```python
from build123d import *

# Parameters (mm, degrees)
SKETCH1_R                = 34.544
BOSS_EXTRUDE1_DEPTH      = 7.62
SKETCH2_R                = 28.1686
CUT_EXTRUDE1_DEPTH       = 3.048
CUT_EXTRUDE2_START       = -1.778
SKETCH3_R                = 28.1686
SKETCH3_R_2              = 4.3688
CUT_EXTRUDE2_DEPTH       = 1.778
CUT_EXTRUDE3_DEPTH       = 50.200658898
FILLET1_R                = 1.6002
CIRPATTERN1_COUNT        = 5
FILLET1_OF_CIRPATTERN1_R = 1.6002
SKETCH5_R                = 17.4625
SKETCH5_R_2              = 10.7061
BOSS_EXTRUDE2_DEPTH      = 1.778
BOSS_EXTRUDE4_START      = 1.6002
SKETCH6_R                = 17.4625
SKETCH6_R_2              = 16.4211
BOSS_EXTRUDE4_DEPTH      = 1.6002
SKETCH7_R                = 3.175
CUT_EXTRUDE4_DEPTH       = 50.066068275
SKETCH8_R                = 1.4224
CUT_EXTRUDE5_DEPTH       = 50.066068275
CIRPATTERN2_COUNT        = 5
BOSS_EXTRUDE5_DEPTH      = 0.0254
BOSS_EXTRUDE5_DEPTH_BACK = 7.6454
SKETCH9_R                = 34.5567
SKETCH9_R_2              = 30.4165
SCALE_1_SCALE            = 3


with BuildPart() as part:
    # Sketch1 → Boss-Extrude1 (new body)
    with BuildSketch(Plane(origin=(0, 0, 0), x_dir=(0, 0, -1), z_dir=(1, 0, 0))):
        with Locations(Location((0, 0, 0), (0, 0, 180))):
            Circle(SKETCH1_R)
    extrude(amount=BOSS_EXTRUDE1_DEPTH)

    # Sketch2 → Cut-Extrude1 (cut)
    with BuildSketch(Plane(origin=(7.62, 0, 0), x_dir=(0, 0, -1), z_dir=(1, 0, 0))):
        Circle(SKETCH2_R)
    extrude(amount=-CUT_EXTRUDE1_DEPTH, mode=Mode.SUBTRACT)

    # Sketch3 → Cut-Extrude2 (cut)
    with BuildSketch(Plane.ZY.offset(CUT_EXTRUDE2_START)):
        with Locations(Location((0, 0, 0), (0, 0, 180))):
            Circle(SKETCH3_R)
        Circle(SKETCH3_R_2, mode=Mode.SUBTRACT)
    extrude(amount=CUT_EXTRUDE2_DEPTH, mode=Mode.SUBTRACT)

    # Sketch4 → Cut-Extrude3 (cut, through all)
    with BuildSketch(Plane.ZY.offset(-1.778)):
        with BuildLine():
            Line((-2.54, 6.985), (2.54, 6.985))
            Line((2.54, 6.985), (9.114287493, 25.064290604))
            ThreePointArc((9.114287493, 25.064290604), (0, 26.67), (-9.114287493, 25.064290604))
            Line((-9.114287493, 25.064290604), (-2.54, 6.985))
        make_face()
    cut_extrude3 = extrude(amount=-CUT_EXTRUDE3_DEPTH, mode=Mode.SUBTRACT)

    # Fillet1
    fillet1_edges = [part.edges().sort_by_distance(p)[0] for p in [
        (3.175, 25.064290604, 9.114287493),
        (3.175, 6.985, 2.54),
        (3.175, 6.985, -2.54),
        (3.175, 25.064290604, -9.114287493),
    ]]
    fillet(fillet1_edges, radius=FILLET1_R)

    # CirPattern1: Cut-Extrude3 ×5 about axis
    cirpattern1_axis = Axis((0, 0, 0), (1, 0, 0))
    for i in range(1, CIRPATTERN1_COUNT):
        add(cut_extrude3.rotate(cirpattern1_axis, i * 360 / CIRPATTERN1_COUNT), mode=Mode.SUBTRACT)

    # Fillet1 of CirPattern1
    fillet1_of_cirpattern1_edges = [part.edges().sort_by_distance(p)[0] for p in [
        (3.175, -0.922910762, 26.654026632),
        (3.175, -0.257199846, 7.428032932),
        (3.175, 4.574167257, 5.858226601),
        (3.175, 16.41349426, 21.021087179),
        (3.175, -25.634680824, 7.358806903),
        (3.175, -7.143958247, 2.050776822),
        (3.175, -4.158009165, 6.160583153),
        (3.175, -14.920193278, 22.10603385),
        (3.175, -14.920193278, -22.10603385),
        (3.175, -4.158009165, -6.160583153),
        (3.175, -7.143958247, -2.050776822),
        (3.175, -25.634680824, -7.358806903),
        (3.175, 16.41349426, -21.021087179),
        (3.175, 4.574167257, -5.858226601),
        (3.175, -0.257199846, -7.428032932),
        (3.175, -0.922910762, -26.654026632),
    ]]
    fillet(fillet1_of_cirpattern1_edges, radius=FILLET1_OF_CIRPATTERN1_R)

    # Sketch5 → Boss-Extrude2 (add)
    with BuildSketch(Plane(origin=(4.572, 0, 0), x_dir=(0, 0, -1), z_dir=(1, 0, 0))):
        Circle(SKETCH5_R)
        Circle(SKETCH5_R_2, mode=Mode.SUBTRACT)
    extrude(amount=-BOSS_EXTRUDE2_DEPTH)

    # Sketch6 → Boss-Extrude4 (add)
    with BuildSketch(Plane(origin=(4.572, 0, 0), x_dir=(0, 0, -1), z_dir=(1, 0, 0)).offset(BOSS_EXTRUDE4_START)):
        Circle(SKETCH6_R)
        Circle(SKETCH6_R_2, mode=Mode.SUBTRACT)
    extrude(amount=-BOSS_EXTRUDE4_DEPTH)

    # Sketch7 → Cut-Extrude4 (cut, through all)
    with BuildSketch(Plane(origin=(4.572, 0, 0), x_dir=(0, 0, -1), z_dir=(1, 0, 0))):
        Circle(SKETCH7_R)
    extrude(amount=-CUT_EXTRUDE4_DEPTH, mode=Mode.SUBTRACT)

    # Sketch8 → Cut-Extrude5 (cut, through all)
    with BuildSketch(Plane(origin=(4.572, 0, 0), x_dir=(0, 0, -1), z_dir=(1, 0, 0))):
        with Locations((0, -6.35)):
            Circle(SKETCH8_R)
    cut_extrude5 = extrude(amount=-CUT_EXTRUDE5_DEPTH, mode=Mode.SUBTRACT)

    # CirPattern2: Cut-Extrude5 ×5 about axis
    cirpattern2_axis = Axis((0, 0, 0), (1, 0, 0))
    for i in range(1, CIRPATTERN2_COUNT):
        add(cut_extrude5.rotate(cirpattern2_axis, i * 360 / CIRPATTERN2_COUNT), mode=Mode.SUBTRACT)

    # Sketch9 → Boss-Extrude5 (add, two sides: drawn at the far end of the back side and taken through both)
    with BuildSketch(Plane(origin=(7.62, 0, 0), x_dir=(0, 0, -1), z_dir=(1, 0, 0)).offset(-BOSS_EXTRUDE5_DEPTH_BACK)):
        Circle(SKETCH9_R)
        Circle(SKETCH9_R_2, mode=Mode.SUBTRACT)
    extrude(amount=BOSS_EXTRUDE5_DEPTH + BOSS_EXTRUDE5_DEPTH_BACK)


with BuildPart() as part_1:
    # 缩放比例1: scaled about (0, 0, 0)
    add(part.part.scale(SCALE_1_SCALE))


solid = part_1.part
```
Could you check a few things on this model? Use its own coordinates, in mm. A direction names the side the tool comes from. Give positions to 0.01 mm unless a question says otherwise; leave off trailing zeros. Order: outer loops, then holes, each group sorted by start corner. A loop starts at its lowest first (then second) coordinate and runs counter-clockwise, first axis right, second up.
Q1. If I drill on line 1 along Y through (x, z) = (16.5, 0); line 2 along Y through (x, z) = (4.25, 0) (3 decimals); line 3 along Y through (x, z) = (11.75, 0) (1 decimal), over which ranges is the centre line in solid material (lowest first)?
Q2. Suppose I cut it at B-B, the plane z = 0. Count the separate pieces of the cut face and the enclosed holes in it, and give its area (3 significant figures).
Q3. I'm going to push flat-ended pins straight in: P1, Ø12, axis at x = 12.5, y = 55, coming from the -Z side; P2, Ø8, axis at y = 12.5, z = -42.5, coming from the -X side; P3, Ø11, axis at y = -19.05, z = 0, coming from the -X side; P4, Ø5, axis at y = -5.89, z = 18.12, coming from the +X side. Where does each tip first touch, or does it pass through?
Q4. For faces 1 (the flat face through (13.716, 1, -10)), 2 (the flat face through (8.5, -53.3, 15.3)), 3 (the flat face through (9, 20.955, 0)), which set-ups out of +Z, -Z, +X, -X, +Y, -Y let a thin tool reach every point of the face, with its end or its side?
Q5. Suppose I cut it at A-A, the plane y = -55.5. Write out the boundary of the cut face in (x, z), and give its area (3 significant figures).
Q6. Suppose I cut it at C-C, the plane y = -81.5. Write out the boundary of the cut face in (x, z), and give its area (3 significant figures).
Q7. We'd pull the mould along Y, two halves only. Please class faces 4 (the flat face through (22.936, -92, 0)), 5 (the cylindrical face through (11.27, -63.08, 82.27)), 6 (the cylindrical face through (9.584, -13.535, -18.459)): +Y half, -Y half, draft (parallel to the pull), parting line (faces both ways), or undercut.
Solution:
1. line 1: y = -103.67 to -84.51, -52.39 to -49.26, 49.26 to 52.39, 84.51 to 103.67
1. line 2: y = -103.67 to -84.506, -13.106 to -9.525, 9.525 to 13.106, 84.506 to 103.67
1. line 3: y = -103.7 to -23.3, -14.8 to -9.5, 9.5 to 21, 32.1 to 52.4, 80 to 103.7
2. separate pieces: 5
2. enclosed holes: 0
2. area: 1,750 mm2
3. P1: stops at z = -91.36
3. P2: stops at x = 8.38
3. P3: stops at x = 5.33
3. P4: passes through
4. face 1: +X
4. face 2: -X
4. face 3: +X, -X
5. outline: (-0.08, -87.56) - (22.94, -87.56) - (22.94, -72.43) - (22.86, -72.43) - (22.86, -63.73) - (13.72, -63.73) - (13.72, -57.63) - (5.33, -57.63) - (5.33, -63.73) - (0, -63.73) - (0, -72.43) - (-0.08, -72.43) - close; (-0.08, 72.43) - (0, 72.43) - (0, 63.73) - (5.33, 63.73) - (5.33, 57.63) - (13.72, 57.63) - (13.72, 63.73) - (22.86, 63.73) - (22.86, 72.43) - (22.94, 72.43) - (22.94, 87.56) - (-0.08, 87.56) - close; (5.33, -15.93) - (13.72, -15.93) - (13.72, 15.93) - (5.33, 15.93) - close
5. area: 1,460 mm2
6. outline: (-0.08, -64.07) - (22.94, -64.07) - (22.94, -41.04) - (22.86, -41.04) - (22.86, -22.34) - (13.72, -22.34) - (13.72, 22.34) - (22.86, 22.34) - (22.86, 41.04) - (22.94, 41.04) - (22.94, 64.07) - (-0.08, 64.07) - (-0.08, 41.04) - (0, 41.04) - (0, 22.34) - (5.33, 22.34) - (5.33, -22.34) - (0, -22.34) - (0, -41.04) - (-0.08, -41.04) - close
6. area: 2,290 mm2
7. face 4: draft
7. face 5: parting line
7. face 6: undercut
